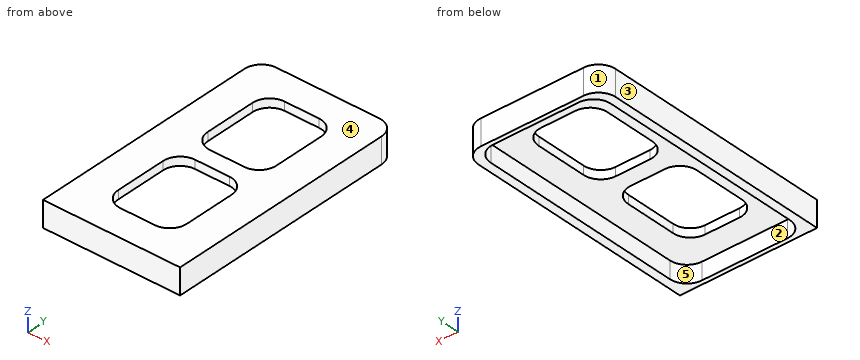
```python
from build123d import *

# Parameters (mm, degrees)
F1_DEPTH = 5
F2_DEPTH = 15


with BuildPart() as f1:
    # F0 (on Top) → F1 (new body)
    with BuildSketch(Plane.XY):
        with BuildLine():
            ThreePointArc((40, 62.5), (37.071068, 69.571068), (30, 72.5))
            Line((30, 72.5), (-30, 72.5))
            ThreePointArc((-30, 72.5), (-37.071068, 69.571068), (-40, 62.5))
            Line((-40, 62.5), (-40, -72.5))
            Line((-40, -72.5), (40, -72.5))
            Line((40, -72.5), (40, 62.5))
        make_face()
        with BuildLine():
            Line((-25, 70), (25, 70))
            ThreePointArc((25, 70), (32.071068, 67.071068), (35, 60))
            Line((35, 60), (35, -60))
            ThreePointArc((35, -60), (32.071068, -67.071068), (25, -70))
            Line((25, -70), (-25, -70))
            ThreePointArc((-25, -70), (-32.071068, -67.071068), (-35, -60))
            Line((-35, -60), (-35, 60))
            ThreePointArc((-35, 60), (-32.071068, 67.071068), (-25, 70))
        make_face(mode=Mode.SUBTRACT)
        with BuildLine():
            ThreePointArc((35, 60), (32.071068, 67.071068), (25, 70))
            Line((25, 70), (-25, 70))
            ThreePointArc((-25, 70), (-32.071068, 67.071068), (-35, 60))
            Line((-35, 60), (-35, -60))
            ThreePointArc((-35, -60), (-32.071068, -67.071068), (-25, -70))
            Line((-25, -70), (25, -70))
            ThreePointArc((25, -70), (32.071068, -67.071068), (35, -60))
            Line((35, -60), (35, 60))
        make_face()
        with BuildLine():
            ThreePointArc((20, -45), (17.071068, -52.071068), (10, -55))
            Line((10, -55), (-10, -55))
            ThreePointArc((-10, -55), (-17.071068, -52.071068), (-20, -45))
            Line((-20, -45), (-20, -15))
            ThreePointArc((-20, -15), (-17.071068, -7.928932), (-10, -5))
            Line((-10, -5), (10, -5))
            ThreePointArc((10, -5), (17.071068, -7.928932), (20, -15))
            Line((20, -15), (20, -45))
        make_face(mode=Mode.SUBTRACT)
        with BuildLine():
            Line((-10, 55), (10, 55))
            ThreePointArc((10, 55), (17.071068, 52.071068), (20, 45))
            Line((20, 45), (20, 15))
            ThreePointArc((20, 15), (17.071068, 7.928932), (10, 5))
            Line((10, 5), (-10, 5))
            ThreePointArc((-10, 5), (-17.071068, 7.928932), (-20, 15))
            Line((-20, 15), (-20, 45))
            ThreePointArc((-20, 45), (-17.071068, 52.071068), (-10, 55))
        make_face(mode=Mode.SUBTRACT)
    extrude(amount=-F1_DEPTH)

    # F0 (on Top) → F2 (join)
    with BuildSketch(Plane.XY):
        with BuildLine():
            ThreePointArc((40, 62.5), (37.071068, 69.571068), (30, 72.5))
            Line((30, 72.5), (-30, 72.5))
            ThreePointArc((-30, 72.5), (-37.071068, 69.571068), (-40, 62.5))
            Line((-40, 62.5), (-40, -72.5))
            Line((-40, -72.5), (40, -72.5))
            Line((40, -72.5), (40, 62.5))
        make_face()
        with BuildLine():
            Line((-25, 70), (25, 70))
            ThreePointArc((25, 70), (32.071068, 67.071068), (35, 60))
            Line((35, 60), (35, -60))
            ThreePointArc((35, -60), (32.071068, -67.071068), (25, -70))
            Line((25, -70), (-25, -70))
            ThreePointArc((-25, -70), (-32.071068, -67.071068), (-35, -60))
            Line((-35, -60), (-35, 60))
            ThreePointArc((-35, 60), (-32.071068, 67.071068), (-25, 70))
        make_face(mode=Mode.SUBTRACT)
    extrude(amount=-F2_DEPTH)


solid = f1.part
```
Geometry check sheet. Reference: the model listing, model coordinates, mm. Face numbers are marked on the shaded views. A direction names the side the tool comes from. Coordinates: 2 decimals unless noted, no trailing zeros. Order: outer loops, then holes, each group sorted by start corner. A loop starts at its lowest first (then second) coordinate and runs counter-clockwise, first axis right, second up.
Item 1: Scan lines: line 1 along X through (y, z) = (20, -1.75); line 2 along X through (y, z) = (-3, -5.75); line 3 along Y through (x, z) = (-17.5, -8.75). Record each from-to range of solid material in increasing order.
Item 2: Section check B-B (z = -12.75). Enter the section's corners in (x, y).
Item 3: Section check D-D (z = -3.5). Enter the section's corners in (x, y).
Item 4: Section check C-C (x = 0). Enter the section's corners in (y, z).
Item 5: Section check A-A (y = -40.5). Enter the section's corners in (x, z).
Item 6: Tool access check on the marked faces 4 and 5. Record the directions out of +Z, -Z, +X, -X, +Y, -Y that give a thin tool (end or side, any length) a straight path to the whole face; none if there is none.
Item 7: Mould release check, pull along Y, two halves, no side actions. Record for the marked faces 1, 2 and 3: released by +Y, released by -Y, zero draft, split by the parting line, or undercut.
Check sheet entries:
1. line 1: x = -40 to -20, 20 to 40
1. line 2: x = -40 to -35, 35 to 40
1. line 3: y = -72.5 to -70, 70 to 72.5
2. outline: (-40, -72.5) - (40, -72.5) - (40, 62.5) arc R10 ccw to (30, 72.5) - (-30, 72.5) arc R10 ccw to (-40, 62.5) - close; hole (-35, -60) arc R10 ccw to (-25, -70) - (25, -70) arc R10 ccw to (35, -60) - (35, 60) arc R10 ccw to (25, 70) - (-25, 70) arc R10 ccw to (-35, 60) - close
3. outline: (-40, -72.5) - (40, -72.5) - (40, 62.5) arc R10 ccw to (30, 72.5) - (-30, 72.5) arc R10 ccw to (-40, 62.5) - close; hole (-20, -45) arc R10 ccw to (-10, -55) - (10, -55) arc R10 ccw to (20, -45) - (20, -15) arc R10 ccw to (10, -5) - (-10, -5) arc R10 ccw to (-20, -15) - close; hole (-20, 15) arc R10 ccw to (-10, 5) - (10, 5) arc R10 ccw to (20, 15) - (20, 45) arc R10 ccw to (10, 55) - (-10, 55) arc R10 ccw to (-20, 45) - close
4. outline: (-72.5, -15) - (-70, -15) - (-70, -5) - (-55, -5) - (-55, 0) - (-72.5, 0) - close; (-5, -5) - (5, -5) - (5, 0) - (-5, 0) - close; (55, -5) - (70, -5) - (70, -15) - (72.5, -15) - (72.5, 0) - (55, 0) - close
5. outline: (-40, -15) - (-35, -15) - (-35, -5) - (-20, -5) - (-20, 0) - (-40, 0) - close; (20, -5) - (35, -5) - (35, -15) - (40, -15) - (40, 0) - (20, 0) - close
6. face 4: +Z, +X, -X, +Y, -Y
6. face 5: -Z
7. face 1: released by +Y
7. face 2: undercut
7. face 3: zero draft
